Verification items for the finished model (mm, model axes). A direction names the side the tool comes from. Round coordinates to 2 decimals unless told otherwise and drop trailing zeros. Write each loop counter-clockwise with the first axis right and the second up, starting at its lowest first coordinate (ties: lowest second). Pieces come first, ordered by that corner, then holes.
from build123d import *

# Parameters (mm, degrees)
F0_W      = 87
F0_H      = 87
F1_DEPTH  = 87
F3_DEPTH  = 43.5
F5_DEPTH  = 43.5
F6_R      = 14.4377052149
F7_DEPTH  = 85
F8_R      = 13.9088324257
F9_DEPTH  = 85
F10_R     = 14.310913908
F11_DEPTH = 87
F13_DEPTH = 43.5
F15_DEPTH = 85
F16_R     = 17.3517727339
F17_DEPTH = 87


with BuildPart() as f1:
    # F0 (on Front) → F1 (new body)
    with BuildSketch(Plane.XZ):
        with Locations((1.9772734489, 0)):
            Rectangle(F0_W, F0_H)
    extrude(amount=F1_DEPTH)

    # F2 (on face) → F3 (cut)
    with BuildSketch(Plane.XY.offset(43.5)):
        Polygon((-41.5227265511, 0), (-41.5227265511, -53.0289933085), (0, -37.420453267), (-4.6001030132, 0), align=None)
    extrude(amount=-F3_DEPTH, mode=Mode.SUBTRACT)

    # F4 (on face) → F5 (cut)
    with BuildSketch(Plane.XZ.offset(87)):
        Polygon((45.4772734489, 43.5), (-12.4589475545, -13.403512232), (16.6048314422, -43.5), (45.4772734489, -43.5), align=None)
    extrude(amount=-F5_DEPTH, mode=Mode.SUBTRACT)

    # F6 (on face) → F7 (cut)
    with BuildSketch(Plane(origin=(0, 0, -43.5), x_dir=(1, 0, 0), z_dir=(0, 0, -1))):
        with Locations((-13.5299172252, 26.452422142)):
            Circle(F6_R)
    extrude(amount=-F7_DEPTH, mode=Mode.SUBTRACT)

    # F8 (on face) → F9 (cut)
    with BuildSketch(Plane(origin=(-41.5227265511, 0, 0), x_dir=(0, -1, 0), z_dir=(-1, 0, 0))):
        with Locations((25.2458769828, -18.6489578336)):
            Circle(F8_R)
    extrude(amount=-F9_DEPTH, mode=Mode.SUBTRACT)

    # F10 (on face) → F11 (cut)
    with BuildSketch(Plane(origin=(0.5832279038, 0, -0.593812568), x_dir=(0.7134366695, 0, 0.7007197147), z_dir=(0.7007197147, 0, -0.7134366695))):
        with Locations((20.3147400171, 65.25)):
            Circle(F10_R)
    extrude(amount=-F11_DEPTH, mode=Mode.SUBTRACT)

    # F12 (on face) → F13 (join)
    with BuildSketch(Plane.XZ.offset(43.5)):
        Polygon((45.4772734489, 3.3152910087), (7.1438206622, -33.7028158401), (12.2559760747, -38.9966189225), (45.4772734489, -6.9152527408), align=None)
    extrude(amount=F13_DEPTH)

    # F14 (on face) → F15 (cut)
    with BuildSketch(Plane(origin=(-41.5227265511, 0, 0), x_dir=(0, -1, 0), z_dir=(-1, 0, 0))):
        with BuildLine():
            ThreePointArc((37.9539034635, -24.3024242405), (57.8630917211, -32.0424114958), (70.742568812, -15.001218766))
            ThreePointArc((70.742568812, -15.001218766), (65.5543826661, -2.4758294084), (53.0289933085, 2.7123567374))
            Line((53.0289933085, 2.7123567374), (53.0289933085, 0))
            Line((53.0289933085, 0), (43.6091104722, 0))
            ThreePointArc((43.6091104722, 0), (38.9372170577, -4.2684372434), (36.0638383113, -9.9066851234))
            ThreePointArc((36.0638383113, -9.9066851234), (38.3592447949, -14.0126657732), (39.1547094085, -18.6489578336))
            ThreePointArc((39.1547094085, -18.6489578336), (38.8511963511, -21.5387509634), (37.9539034635, -24.3024242405))
        make_face()
        with BuildLine():
            Line((53.0289933085, 0), (53.0289933085, 2.7123567374))
            ThreePointArc((53.0289933085, 2.7123567374), (48.1276906317, 2.0207666994), (43.6091104722, 0))
            Line((43.6091104722, 0), (53.0289933085, 0))
        make_face()
    extrude(amount=-F15_DEPTH, mode=Mode.SUBTRACT)

    # F16 (on face) → F17 (cut)
    with BuildSketch(Plane(origin=(12.3249261037, -32.7874698726, 0), x_dir=(-0.9360508251, -0.3518648219, 0), z_dir=(-0.3518648219, 0.9360508251, 0))):
        with Locations((33.5201099515, 23.305317387)):
            Circle(F16_R)
    extrude(amount=-F17_DEPTH, mode=Mode.SUBTRACT)


solid = f1.part
Q1. Sectioned sample at A-A (z = -28.5). Enter the section's corners in (x, y), plus the area to 3 significant figures.
Recorded:
outline: (-41.52, -87) - (2.12, -87) - (2.12, -64.5) - (-41.52, -64.5) - close; (-41.52, -41.56) - (43.48, -41.56) - (43.48, -43.5) - (45.48, -43.5) - (45.48, 0) - (-41.52, 0) - (-41.52, -15.43) - (-22.85, -15.43) arc R14.44 cw to (-4.21, -15.43) - (43.48, -15.43) - (43.48, -35.06) - (-1.94, -35.06) arc R14.44 cw to (-25.12, -35.06) - (-41.52, -35.06) - close; (12.53, -87) - (23.13, -87) - (23.13, -64.5) - (12.53, -64.5) - close
area: 3,030 mm2
Q2. Sectioned sample at D-D (x = -14). Give the number of separate pieces and of enclosed holes in the cut face, plus the area to 3 significant figures.
Recorded:
separate pieces: 4
enclosed holes: 0
area: 2,000 mm2
Q3. Tool access check on faces 5 (the cylindrical face through (-0.037, -21.316, 7.233)), 6 (the flat face through (43.477, -34, -15)), 7 (the flat face through (-0.617, -75.221, -25.667)), 8 (the flat face through (14.4, -65.554, -41.217)). Record the directions out of +Z, -Z, +X, -X, +Y, -Y that give a thin tool (end or side, any length) a straight path to the whole face; none if there is none.
Recorded:
face 5: -Z
face 6: -X
face 7: -Y
face 8: +X, -Y
Q4. Material ranges on line 1 along Z through (x, y) = (15.5, -63); line 2 along Z through (x, y) = (-24, -54); line 3 along X through (y, z) = (-14, -23), recorded low to high.
Recorded:
line 1: z = -43.5 to -42.36, -35.86 to -29.64, 33.38 to 43.5
line 2: z = -43.5 to -32.69, 2.69 to 7.88, 38.73 to 40.8
line 3: x = 43.48 to 45.48
Q5. Release check for a two-part mould opening along X. For faces 1 (the flat face through (7, -43.5, -31)), 2 (the flat face through (26.579, -74.612, -14.935)), 3 (the flat face through (-34.893, -50.537, 17.221)), 4 (the flat face through (24.94, -74.61, -26.75)) record: released by +X, released by -X, zero draft, split by the parting line, or undercut.
Recorded:
face 1: undercut
face 2: undercut
face 3: released by -X
face 4: released by +X
Q6. Sectioned sample at B-B (x = 40). Enter the section's corners in (y, z), plus the area to 3 significant figures.
Recorded:
outline: (-87, -12.2) - (-70.52, -12.2) arc R17.71 cw to (-65.03, -1.97) - (-87, -1.97) - close; (-87, 38.12) - (-43.5, 38.12) - (-43.5, -0.07) arc R17.71 cw to (-36.06, -9.91) arc R13.91 cw (long way) to (-37.95, -24.3) arc R17.71 cw to (-43.5, -29.93) - (-43.5, -43.5) - (0, -43.5) - (0, 43.5) - (-87, 43.5) - close
area: 3,460 mm2
Q7. Depth check by flat-ended pin: P1, Ø1, axis at y = -71.5, z = -13.5, coming from the +X side; P2, Ø3, axis at x = 31, z = 17, coming from the -Y side; P3, Ø1.5, axis at x = -1, z = -15, coming from the -Y side. Enter the tip coordinate at first touch or a pass-through.
Recorded:
P1: stops at x = 39.18
P2: stops at y = -43.5
P3: stops at y = -12.05
Q8. Sectioned sample at C-C (x = 31). Enter the section's corners in (y, z).
Recorded:
outline: (-87, -20.9) - (-69.73, -20.9) arc R17.71 cw to (-70.2, -10.67) - (-87, -10.67) - close; (-87, 29.28) - (-43.5, 29.28) - (-43.5, -0.07) arc R17.71 cw to (-36.06, -9.91) arc R13.91 cw (long way) to (-37.95, -24.3) arc R17.71 cw to (-43.5, -29.93) - (-43.5, -43.5) - (0, -43.5) - (0, 43.5) - (-87, 43.5) - close
